Build history of the part. All positions in model axes, mm. A direction names the side the tool comes from. Give positions to 0.01 mm unless a question says otherwise; leave off trailing zeros. Order: outer loops, then holes, each group sorted by start corner. A loop starts at its lowest first (then second) coordinate and runs counter-clockwise, first axis right, second up. Notation, with made-up numbers: (-6.75, 2.5) -> (1.25, 2.5) arc R21 ccw to (1.25, 29.5) -> close; hole circle Ø5 at (-32.5, -35). An arc over 180 degrees is marked (long way). One line per question, with ' | ' between items. Start each with the question number.
(1) Cut at B-B (z = 1.25). Give the cut face in (x, y), then the cut area to 3 significant figures.
(2) Drill centre lines: L1, parallel to Y at x = -6.5, z = 9; L2, parallel to Z at x = -15.5, y = -5.5; L3, parallel to X at y = 0.5, z = 2.25. Where is each one in solid material? Low to high. Write a range as from..to.
(3) Which spindle directions (+Z, -Z, +X, -X, +Y, -Y) get a long thin tool onto all of the face, cutting with end or side? Do faces 4 (the face through (-20.07, -10.377, 6.783)), 5 (the face through (-3, 5.55, 6)), 6 (the face through (-3, -5.55, 6)), 7 (the face through (21.295, -0.279, 8.549)). Say none if no direction does.
(4) Pull direction Z, two halves, no side cores. Call faces 1 (the face through (-20.07, -0.14, 2.23)), 2 (the face through (-2, 3.5, 9)), 3 (the face through (8, 0, 5)): +Z half, -Z half, draft (parallel to the pull), parting line (faces both ways), or undercut.
(5) Cut at D-D (y = -0.5). Give the cut face in (x, z), then the cut area to 3 significant figures.
(6) Cut at A-A (z = 6.5). Give the cut face in (x, y).
(7) Cut at C-C (x = -1.5). Give the cut face in (y, z).
(8) Pin check, flat tips, straight feed: pin 1 Ø5 at (x, y) = (10, 1) entering from +Z; pin 2 Ø2 at (y, z) = (5.5, 5.5) entering from +X; pin 3 Ø1.8 at (x, z) = (-22, 6.5) entering from +Y; pin 4 Ø2 at (y, z) = (4, 4.5) entering from +X. Stop position of each tip, or through.
from build123d import *

# Parameters (mm, degrees)
SKETCH1_W           = 50
SKETCH1_H           = 30
BOSS_EXTRUDE1_DEPTH = 15
SKETCH2_R           = 4.5
CUT_EXTRUDE1_DEPTH  = 10
SKETCH4_R           = 7.5
CUT_EXTRUDE3_DEPTH  = 10
SKETCH5_R           = 1.25
CUT_EXTRUDE4_DEPTH  = 10
SKETCH7_W           = 50
SKETCH7_H           = 30
CUT_EXTRUDE5_DEPTH  = 3
CUT_EXTRUDE6_DEPTH  = 13
SKETCH9_R           = 1.5
CUT_EXTRUDE7_DEPTH  = 23


with BuildPart() as part:
    # Sketch1 → Boss-Extrude1 (new body)
    with BuildSketch(Plane.XY):
        Rectangle(SKETCH1_W, SKETCH1_H)
    extrude(amount=BOSS_EXTRUDE1_DEPTH)

    # Sketch2 → Cut-Extrude1 (cut)
    with BuildSketch(Plane.ZY.offset(25)):
        with Locations((6.728688525, -0.205173042)):
            Circle(SKETCH2_R)
        with BuildLine():
            Line((9.178688525, 7.516794171), (9.178688525, -7.927140255))
            ThreePointArc((9.178688525, -7.927140255), (6.728688525, -10.377140255), (4.278688525, -7.927140255))
            Line((4.278688525, -7.927140255), (4.278688525, 7.516794171))
            ThreePointArc((4.278688525, 7.516794171), (6.728688525, 9.966794171), (9.178688525, 7.516794171))
        make_face()
    extrude(amount=-CUT_EXTRUDE1_DEPTH, mode=Mode.SUBTRACT)

    # Sketch4 → Cut-Extrude3 (cut)
    with BuildSketch(Plane.XY.offset(15)):
        with Locations((13.8, 0)):
            Circle(SKETCH4_R)
        with BuildLine():
            Line((-10, 3.5), (13.8, 3.5))
            ThreePointArc((13.8, 3.5), (17.3, 0), (13.8, -3.5))
            Line((13.8, -3.5), (-10, -3.5))
            ThreePointArc((-10, -3.5), (-13.5, 0), (-10, 3.5))
        make_face()
    extrude(amount=-CUT_EXTRUDE3_DEPTH, mode=Mode.SUBTRACT)

    # Sketch5 → Cut-Extrude4 (cut)
    with BuildSketch(Plane.XY.offset(5)):
        with Locations((-10.053055142, 0)):
            Circle(SKETCH5_R)
        with Locations((-6.053055142, 0)):
            Circle(SKETCH5_R)
    extrude(amount=-CUT_EXTRUDE4_DEPTH, mode=Mode.SUBTRACT)

    # Sketch7 → Cut-Extrude5 (cut)
    with BuildSketch(Plane.XY.offset(15)):
        Rectangle(SKETCH7_W, SKETCH7_H)
    extrude(amount=-CUT_EXTRUDE5_DEPTH, mode=Mode.SUBTRACT)

    # Sketch8 → Cut-Extrude6 (cut)
    with BuildSketch(Plane.XY.offset(12)):
        with BuildLine():
            Line((-25, 15), (-25, 10.92225852))
            Line((-25, 10.92225852), (-16.637103876, 10.92225852))
            Line((-16.637103876, 10.92225852), (-11.26502882, 5.550183464))
            Line((-11.26502882, 5.550183464), (5.459842894, 5.550183464))
            ThreePointArc((5.459842894, 5.550183464), (23.343165243, 0), (5.459842894, -5.550183464))
            Line((5.459842894, -5.550183464), (-11.26502882, -5.550183464))
            Line((-11.26502882, -5.550183464), (-16.637103876, -10.92225852))
            Line((-16.637103876, -10.92225852), (-25, -10.92225852))
            Line((-25, -10.92225852), (-25, -15))
            Line((-25, -15), (25, -15))
            Line((25, -15), (25, 15))
            Line((25, 15), (-25, 15))
        make_face()
    extrude(amount=-CUT_EXTRUDE6_DEPTH, mode=Mode.SUBTRACT)

    # Sketch9 → Cut-Extrude7 (cut)
    with BuildSketch(Plane(origin=(0, 10.92225852, 0), x_dir=(1, 0, 0), z_dir=(0, 1, 0))):
        with Locations((-22, -6.5)):
            Circle(SKETCH9_R)
    extrude(amount=-CUT_EXTRUDE7_DEPTH, mode=Mode.SUBTRACT)


solid = part.part
Result set:
1) outline: (-25, -10.92) -> (-16.64, -10.92) -> (-11.27, -5.55) -> (5.46, -5.55) arc R9.8 ccw (long way) to (5.46, 5.55) -> (-11.27, 5.55) -> (-16.64, 10.92) -> (-25, 10.92) -> close; hole circle Ø2.5 at (-10.05, 0); hole circle Ø2.5 at (-6.05, 0) | area: 736 mm2
2) L1: y = -5.55..-3.5, 3.5..5.55 | L2: z = 0..4.28, 9.18..12 | L3: x = -25..-11.2, -8.91..-7.2, -4.91..23.33
3) face 4: -X | face 5: +Z, -Z, +Y | face 6: +Z, -Z, -Y | face 7: +Z
4) face 1: undercut | face 2: draft | face 3: +Z half
5) outline: (-25, 0) -> (-11.2, 0) -> (-11.2, 5) -> (-13.46, 5) -> (-13.46, 12) -> (-25, 12) -> (-25, 11.22) -> (-15, 11.22) -> (-15, 2.24) -> (-25, 2.24) -> close; (-8.91, 0) -> (-7.2, 0) -> (-7.2, 5) -> (-8.91, 5) -> close; (-4.91, 0) -> (23.33, 0) -> (23.33, 12) -> (21.28, 12) -> (21.28, 5) -> (-4.91, 5) -> close | area: 224 mm2
6) outline: (-25, -10.92) -> (-23.5, -10.92) -> (-23.5, -10.37) -> (-25, -10.37) -> close; (-25, 9.96) -> (-23.5, 9.96) -> (-23.5, 10.92) -> (-25, 10.92) -> close; (-20.5, -10.92) -> (-16.64, -10.92) -> (-16.08, -10.37) -> (-20.5, -10.37) -> close; (-20.5, 9.96) -> (-15.67, 9.96) -> (-16.64, 10.92) -> (-20.5, 10.92) -> close; (-15, -9.29) -> (-11.27, -5.55) -> (5.46, -5.55) arc R9.8 ccw (long way) to (5.46, 5.55) -> (-11.27, 5.55) -> (-15, 9.29) -> close; hole (-10, -3.5) -> (7.17, -3.5) arc R7.5 ccw (long way) to (7.17, 3.5) -> (-10, 3.5) arc R3.5 ccw to start
7) outline: (-5.55, 0) -> (5.55, 0) -> (5.55, 12) -> (3.5, 12) -> (3.5, 5) -> (-3.5, 5) -> (-3.5, 12) -> (-5.55, 12) -> close
8) pin 1: stops at z = 5 | pin 2: stops at x = 22.25 | pin 3: passes through | pin 4: stops at x = 22.87
